For this review, take the finished solid that the model builds, in its own axes (mm). Round coordinates to 2 decimals unless told otherwise and drop trailing zeros. Loops run counter-clockwise (first coordinate to the right, second up) from the corner with the lowest first, then second, coordinate; pieces in that order, holes last.
```python
from build123d import *

# Parameters (mm, degrees)
BOSS_EXTRUDE1_DEPTH = 3


with BuildPart() as part:
    # Sketch2 → Boss-Extrude1 (new body)
    with BuildSketch(Plane(origin=(0, 0, 0), x_dir=(1, 0, 0), z_dir=(0, 1, 0))):
        Polygon((-122.911356388, -52), (-128.911356388, -52), (-128.911356388, -26), (-122.911356388, -26), (-122.911356388, 0), (-128.911356388, 0), (-128.911356388, 26), (-122.911356388, 26), (-122.911356388, 52), (-128.911356388, 52), (-128.911356388, 78), (-122.911356388, 78), (-102.911356388, 78), (-102.911356388, 84), (-82.911356388, 84), (-82.911356388, 78), (-62.911356388, 78), (-62.911356388, 84), (53.188643612, 84), (53.188643612, 78), (79.188643612, 78), (79.188643612, 52), (73.188643612, 52), (73.188643612, 26), (79.188643612, 26), (79.188643612, 0), (73.188643612, 0), (73.188643612, -26), (79.188643612, -26), (79.188643612, -52), (73.188643612, -52), (53.188643612, -52), (53.188643612, -58), (-62.911356388, -58), (-62.911356388, -52), (-82.911356388, -52), (-82.911356388, -58), (-102.911356388, -58), (-102.911356388, -52), align=None)
    extrude(amount=BOSS_EXTRUDE1_DEPTH)


solid = part.part
```
(1) For L1, parallel to X at y = 2.65, z = -46; L2, parallel to Z at x = -79.5, y = 2.05, list the stretches that pass through material, from the lowest coordinate up.
(2) Insertion check: pin 1 Ø1.5 at (y, z) = (0.5, -46.5) entering from -X; pin 2 Ø0.9 at (y, z) = (1.5, 12) entering from +X; pin 3 Ø1.5 at (y, z) = (1.5, -82) entering from +X. Each pin has a flat end and moves straight along its axis. Give the tip position at first contact, or say it passes through.
(3) Add section A-A (z = -39.5). Give the boundary of the cut face in (x, y).
Outcome:
1. L1: x = -122.91 to 73.19
1. L2: z = -78 to 52
2. pin 1: stops at x = -122.91
2. pin 2: stops at x = 73.19
2. pin 3: stops at x = 53.19
3. outline: (-122.91, 0) - (73.19, 0) - (73.19, 3) - (-122.91, 3) - close
